For this review, take the finished solid that the model builds, in its own axes (mm). Face numbers are marked on the shaded views. A direction names the side the tool comes from. Give positions to 0.01 mm unless a question says otherwise; leave off trailing zeros. Loops run counter-clockwise (first coordinate to the right, second up) from the corner with the lowest first, then second, coordinate; pieces in that order, holes last.
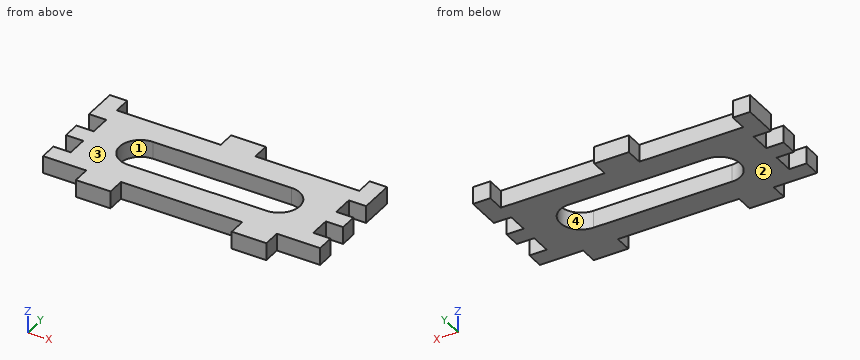
```python
from build123d import *

# Parameters (mm, degrees)
ESQUISSE1_W        = 80
ESQUISSE1_H        = 27
BOSS_EXTRU_1_DEPTH = 5
ESQUISSE3_W        = 5
ESQUISSE3_H        = 6
CR_NEAUX_DEPTH     = 5
ESQUISSE2_W        = 5
ESQUISSE2_H        = 5
ESQUISSE2_W_2      = 10
CR_NEAUX_2_DEPTH   = 5


with BuildPart() as part:
    # Esquisse1 → Boss.-Extru.1 (new body)
    with BuildSketch(Plane.XY):
        with Locations((98.983627477, 156.921111622)):
            Rectangle(ESQUISSE1_W, ESQUISSE1_H)
    extrude(amount=-BOSS_EXTRU_1_DEPTH)

    # Esquisse3 → Cr_neaux (cut)
    with BuildSketch(Plane.XY):
        with Locations((61.483627477, 162.421111622)):
            Rectangle(ESQUISSE3_W, ESQUISSE3_H)
        with Locations((61.483627477, 151.421111622)):
            Rectangle(ESQUISSE3_W, ESQUISSE3_H)
        with Locations((136.483627477, 151.421111622)):
            Rectangle(ESQUISSE3_W, ESQUISSE3_H)
        with Locations((136.483627477, 162.421111622)):
            Rectangle(ESQUISSE3_W, ESQUISSE3_H)
        with BuildLine():
            Line((78.983627477, 162.921111622), (118.983627477, 162.921111622))
            ThreePointArc((118.983627477, 162.921111622), (124.983627477, 156.921111622), (118.983627477, 150.921111622))
            Line((118.983627477, 150.921111622), (78.983627477, 150.921111622))
            ThreePointArc((78.983627477, 150.921111622), (72.983627477, 156.921111622), (78.983627477, 162.921111622))
        make_face()
    extrude(amount=-CR_NEAUX_DEPTH, mode=Mode.SUBTRACT)

    # Esquisse2 → Cr_neaux 2 (add)
    with BuildSketch(Plane.XY):
        with Locations((136.483627477, 172.921111622)):
            Rectangle(ESQUISSE2_W, ESQUISSE2_H)
        with Locations((61.483627477, 172.921111622)):
            Rectangle(ESQUISSE2_W, ESQUISSE2_H)
        with Locations((98.983627477, 172.921111622)):
            Rectangle(ESQUISSE2_W_2, ESQUISSE2_H)
        with Locations((121.483627477, 140.921111622)):
            Rectangle(ESQUISSE2_W_2, ESQUISSE2_H)
        with Locations((76.483627477, 140.921111622)):
            Rectangle(ESQUISSE2_W_2, ESQUISSE2_H)
    extrude(amount=-CR_NEAUX_2_DEPTH)


solid = part.part
```
Q1. Consider section A-A on x = 97.5. Give the boundary of the cut face in (y, z).
Answers:
outline: (143.42, -5) - (150.92, -5) - (150.92, 0) - (143.42, 0) - close; (162.92, -5) - (175.42, -5) - (175.42, 0) - (162.92, 0) - close
Q2. Consider section C-C on x = 70. Give the boundary of the cut face in (y, z).
Answers:
outline: (143.42, -5) - (170.42, -5) - (170.42, 0) - (143.42, 0) - close
Q3. For probe 1 along X at (y, z) = (170.5, -3.2); probe 2 along Y at (x, z) = (114, -1.05); probe 3 along Y at (x, z) = (119, -3.9), list the stretches that pass through material, from the lowest coordinate up.
Answers:
probe 1: x = 58.98 to 63.98, 93.98 to 103.98, 133.98 to 138.98
probe 2: y = 143.42 to 150.92, 162.92 to 170.42
probe 3: y = 138.42 to 150.92, 162.92 to 170.42
Q4. Consider section D-D on y = 164. Give the boundary of the cut face in (x, z), plus the area to 3 significant figures.
Answers:
outline: (63.98, -5) - (133.98, -5) - (133.98, 0) - (63.98, 0) - close
area: 350 mm2
Q5. Mouldability with a two-part tool opening along Y and no side actions: class the marked faces 3 and 4 as +Y half, -Y half, draft (parallel to the pull), parting line (faces both ways), or undercut.
Answers:
face 3: draft
face 4: undercut
Q6. Consider section B-B on y = 156.5. Give the boundary of the cut face in (x, z), plus the area to 3 significant figures.
Answers:
outline: (58.98, -5) - (73, -5) - (73, 0) - (58.98, 0) - close; (124.97, -5) - (138.98, -5) - (138.98, 0) - (124.97, 0) - close
area: 140 mm2
Q7. Machinability: for the marked faces 1 and 2, which of the approach directions +Z, -Z, +X, -X, +Y, -Y give a long, thin tool a straight path to every point of the face, cutting with its end or side? Answer none if there is none.
Answers:
face 1: +Z, -Z
face 2: -Z, +X, -X, +Y, -Y
Q8. For pin 1 Ø1.5 at (x, z) = (126.5, -3) entering from +Y; pin 2 Ø1.5 at (x, z) = (137, -2.5) entering from -Y; pin 3 Ø2.5 at (y, z) = (152.5, -2) entering from +X, all flat-tipped, find the tip position at first contact; note any pin that passes through.
Answers:
pin 1: stops at y = 170.42
pin 2: stops at y = 143.42
pin 3: stops at x = 133.98
